from build123d import *

# Parameters (mm, degrees)
BASPROSKE_W         = 4.55
BASPROSKE_H         = 12
TOOTHCUT_DEPTH      = 18.569931702
TEETHCUTS_COUNT     = 22
TEETHCUTS_ANGLE     = 343.636363636
BORSKE_R            = 1.35
BORE_DEPTH          = 50.0000508
SKETCH1_R           = 4
SKETCH1_R_2         = 1.35
BOSS_EXTRUDE1_DEPTH = 4
SKETCH1_4_R         = 6
SKETCH1_4_R_2       = 4
BOSS_EXTRUDE2_DEPTH = 1
SKETCH2_2_R         = 2.35
CUT_EXTRUDE1_DEPTH  = 3


with BuildPart() as part:
    # BasProSke → Base-Revolve (revolve)
    with BuildSketch(Plane(origin=(0, 0, 0), x_dir=(1, 0, 0), z_dir=(0, 1, 0)), mode=Mode.PRIVATE) as base_revolve_sk:
        with Locations((2.275, 6)):
            Rectangle(BASPROSKE_W, BASPROSKE_H)
    revolve(base_revolve_sk.sketch.rotate(Axis((-10, 0, 0), (1, 0, 0)), 180), axis=Axis((-10, 0, 0), (1, 0, 0)))

    # TooCutSke → ToothCut (cut, through all)
    with BuildSketch(Plane(origin=(0, 0, 0), x_dir=(0, 0, -1), z_dir=(1, 0, 0))):
        with BuildLine():
            ThreePointArc((0.491001901, 9.736627657), (0, 9.749), (-0.491001901, 9.736627657))
            ThreePointArc((-0.491001901, 9.736627657), (-0.822824844, 10.904005344), (-1.46093845, 11.936327074))
            ThreePointArc((-1.46093845, 11.936327074), (0, 12.0254), (1.46093845, 11.936327074))
            ThreePointArc((1.46093845, 11.936327074), (0.822824844, 10.904005344), (0.491001901, 9.736627657))
        make_face()
    toothcut = extrude(amount=TOOTHCUT_DEPTH, mode=Mode.SUBTRACT)

    # TeethCuts: ToothCut ×22 about axis
    teethcuts_axis = Axis((-10, 0, 0), (1, 0, 0))
    for i in range(1, TEETHCUTS_COUNT):
        add(toothcut.rotate(teethcuts_axis, i * TEETHCUTS_ANGLE / (TEETHCUTS_COUNT - 1)), mode=Mode.SUBTRACT)

    # BorSke → Bore (cut, symmetric)
    with BuildSketch(Plane(origin=(0, 0, 0), x_dir=(0, 0, -1), z_dir=(1, 0, 0))):
        with Locations(Location((0, 0, 0), (0, 0, 180))):
            Circle(BORSKE_R)
    extrude(amount=BORE_DEPTH, both=True, mode=Mode.SUBTRACT)

    # Sketch1 → Boss-Extrude1 (add)
    with BuildSketch(Plane.ZY):
        with Locations(Location((0, 0, 0), (0, 0, 180))):
            Circle(SKETCH1_R)
        Circle(SKETCH1_R_2, mode=Mode.SUBTRACT)
    extrude(amount=BOSS_EXTRUDE1_DEPTH)

    # Sketch1_4 → Boss-Extrude2 (add)
    with BuildSketch(Plane.ZY):
        with Locations(Location((0, 0, 0), (0, 0, 180))):
            Circle(SKETCH1_4_R)
        Circle(SKETCH1_4_R_2, mode=Mode.SUBTRACT)
    extrude(amount=BOSS_EXTRUDE2_DEPTH)

    # Sketch2_2 → Cut-Extrude1 (cut)
    with BuildSketch(Plane(origin=(4.55, 0, 0), x_dir=(0, 0, -1), z_dir=(1, 0, 0))):
        Circle(SKETCH2_2_R)
    extrude(amount=-CUT_EXTRUDE1_DEPTH, mode=Mode.SUBTRACT)


solid = part.part
The listing builds one solid part. Answer for the finished solid, in the listing's coordinates (mm). A direction names the side the tool comes from. Give positions to 0.01 mm unless a question says otherwise; leave off trailing zeros. Loops run counter-clockwise (first coordinate to the right, second up) from the corner with the lowest first, then second, coordinate; pieces in that order, holes last. Notation, with made-up numbers: (50, 54.5) - (73, 54.5) arc R16 cw to (73, 68.5) - close; hole circle Ø3 at (2.5, 44.25). An arc over 180 degrees is marked (long way). Answer as a JSON object with one key per item and string values.
1. For faces 1 (the cylindrical face through (2.24, 10.87, 0.81)), 2 (the cylindrical face through (2.24, -8.73, 6.59)), 3 (the cylindrical face through (2.24, -5.28, -9.58)), 4 (the cylindrical face through (2.24, -6.52, 8.78)), determine the directions among +Z, -Z, +X, -X, +Y, -Y from which every point of the face is accessible in a straight line to the end or side of a thin tool.
Determined:
{"face 1": "+X, -X, +Y", "face 2": "+X, -X, -Y", "face 3": "-Z, +X, -X", "face 4": "+X, -X"}
2. Find the intervals of material crossed by L1, parallel to Y at x = -2.05, z = 0; L2, parallel to X at y = 7.75, z = -2.75; L3, parallel to Y at x = 3.25, z = -3.5, in increasing order. Write a range as [from, to].
Determined:
{"L1": "[-4, -1.35], [1.35, 4]", "L2": "[0, 4.55]", "L3": "[-9.74, 9.74]"}
3. A cutting plane is placed at A-A (z = 0). Write down the section's boundary in (x, y).
Determined:
{"outline": "(-4, -4) - (-1, -4) - (-1, -6) - (0, -6) - (0, -9.75) - (4.55, -9.75) - (4.55, -2.35) - (1.55, -2.35) - (1.55, -1.35) - (-4, -1.35) - close; (-4, 1.35) - (1.55, 1.35) - (1.55, 2.35) - (4.55, 2.35) - (4.55, 9.75) - (0, 9.75) - (0, 6) - (-1, 6) - (-1, 4) - (-4, 4) - close"}
4. A cutting plane is placed at B-B (x = -2.25). Write down the section's boundary in (y, z).
Determined:
{"outline": "circle Ø8 at (0, 0); hole circle Ø2.7 at (0, 0)"}
5. For a pull along Z with two mould halves and no side action, classify faces 5 (the cylindrical face through (3.071, -2.294, 0.509)), 6 (the cylindrical face through (-2.479, 3.905, 0.867)), 7 (the cylindrical face through (2.243, -5.254, 9.556)) as pulls with the +Z half, pulls with the -Z half, needs draft (parallel to the pull), parting line crosses it, or undercut.
Determined:
{"face 5": "undercut", "face 6": "parting line crosses it", "face 7": "pulls with the +Z half"}
6. Flat-ended cylindrical pins translate along their axes: pin 1 Ø5 at (y, z) = (-3, 9) entering from -X; pin 2 Ø1.4 at (y, z) = (1, -1) entering from +X; pin 3 Ø1.5 at (x, z) = (3, -3.5) entering from -Y. Find the tip coordinate at first contact, or state that the pin passes through.
Determined:
{"pin 1": "x = 0", "pin 2": "x = 1.55", "pin 3": "y = -10.64"}
